```python
from build123d import *

# Parameters (mm, degrees)
F0_R     = 3.4036
F1_DEPTH = 3.9878
F2_R     = 3.302
F3_DEPTH = 10.16


# Not quite as in the source:
# - a fillet or chamfer that OpenCascade refuses, or shapes differently, is made with other operations: its cross-section is extruded or revolved along the edge and cut away or added


with BuildPart() as f1:
    # F0 (on Top) → F1 (new body)
    with BuildSketch(Plane.XY):
        Circle(F0_R)
    extrude(amount=F1_DEPTH)

    # F2 (on face) → F3 (join)
    with BuildSketch(Plane.XY.offset(3.9878)):
        Circle(F2_R)
    extrude(amount=F3_DEPTH)

    # F4: fillet of radius 1.27 on 2 edges, made by hand

    # F4_s1 → F4_t2 (revolve)
    with BuildSketch(Plane.XZ):
        with BuildLine():
            ThreePointArc((3.4036, 3.9878), (3.3276592107, 4.2315363157), (3.302, 4.4855363157))
            Line((3.302, 4.4855363157), (3.302, 3.9878))
            Line((3.302, 3.9878), (3.4036, 3.9878))
        make_face()
    revolve(axis=Axis((0, 0, 3.9878), (0, 0, 1)))

    # F4_s3 → F4_t4 (revolve, cut)
    with BuildSketch(Plane.XZ):
        with BuildLine():
            ThreePointArc((3.302, 12.8778), (2.9300256121, 13.7758256121), (2.032, 14.1478))
            Line((2.032, 14.1478), (3.302, 14.1478))
            Line((3.302, 14.1478), (3.302, 12.8778))
        make_face()
    revolve(axis=Axis((0, 0, 14.1478), (0, 0, 1)), mode=Mode.SUBTRACT)


solid = f1.part
```
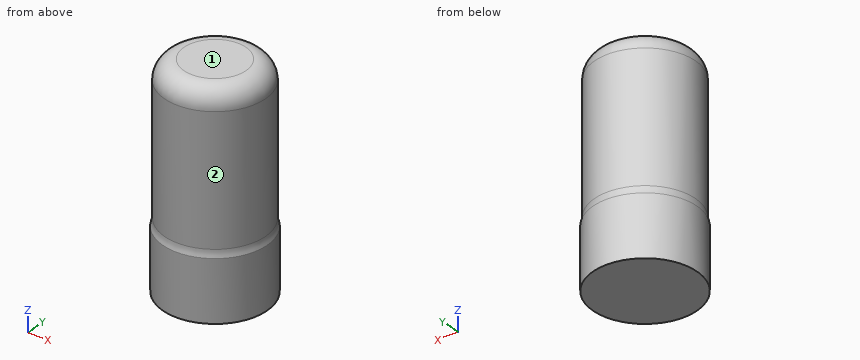
Input: part model. Units: mm. Frame: model coordinates. Face numbers are marked on the shaded views. A direction names the side the tool comes from. Give positions to 0.01 mm unless a question says otherwise; leave off trailing zeros. Loops run counter-clockwise (first coordinate to the right, second up) from the corner with the lowest first, then second, coordinate; pieces in that order, holes last.
1) Section query C-C on z = 6.5. Return the cut outline in (x, y), and give its area (3 significant figures).
A:
outline: circle Ø6.6 at (0, 0)
area: 34.3 mm2
2) Reachability of the marked faces 1 and 2 from +Z, -Z, +X, -X, +Y, -Y: full face, straight path, thin tool, end or side. Return the list, or none.
A:
face 1: +Z, +X, -X, +Y, -Y
face 2: +Z
3) Line query: L1, parallel to X at y = -0.25, z = 13.25; L2, parallel to Z at x = -2, y = -2; L3, parallel to Y at x = -2, z = 5.5. Output: solid intervals per line, ascending.
A:
L1: x = -3.24 to 3.24
L2: z = 0 to 13.87
L3: y = -2.63 to 2.63
4) Contact query for flat-ended pins moving along their axis: pin 1 (3 mm diameter, centred on y = -1.5, z = 2.5, fed in from -X); pin 2 (4 mm diameter, centred on y = 2, z = 11.5, fed in from -X); pin 3 (1.5 mm diameter, centred on x = -1.5, z = 3.5, fed in from -Y). Output: stop coordinate, or through.
A:
pin 1: stops at x = -3.4
pin 2: stops at x = -3.3
pin 3: stops at y = -3.32
5) Section query A-A on x = 0. Return the cut outline in (y, z), and give its area (3 significant figures).
A:
outline: (-3.4, 0) - (3.4, 0) - (3.4, 3.99) arc R1.27 cw to (3.3, 4.49) - (3.3, 12.88) arc R1.27 ccw to (2.03, 14.15) - (-2.03, 14.15) arc R1.27 ccw to (-3.3, 12.88) - (-3.3, 4.49) arc R1.27 cw to (-3.4, 3.99) - close
area: 93.6 mm2
6) Section query D-D on z = 2. Return the cut outline in (x, y), and give its area (3 significant figures).
A:
outline: circle Ø6.81 at (0, 0)
area: 36.4 mm2
